Input: part model. Units: mm. Frame: model coordinates. A direction names the side the tool comes from. Give positions to 0.01 mm unless a question says otherwise; leave off trailing zeros. Order: outer loops, then holes, each group sorted by start corner. A loop starts at its lowest first (then second) coordinate and runs counter-clockwise, first axis right, second up. Notation, with made-up numbers: M 79,41 L 91,41 A16 ccw 91,66 Z; hole C 67,12.25 d6. An arc over 180 degrees is marked long. Use a Markdown table: item, result.
Autodesk Inventor part; units mm, degrees
ref_plane "YZ Plane" through (0, 0, 0) normal (1, 0, 0) x (0, 1, 0)
ref_plane "XZ Plane" through (0, 0, 0) normal (0, 1, 0) x (-1, 0, 0)
ref_plane "XY Plane" through (0, 0, 0) normal (0, 0, 1) x (1, 0, 0)
sketch "main" plane through (0, 0, 0) normal (0, 0, 1) x (1, 0, 0)
  circle A0 centre (13.5257, -15.1463) radius 2.1844
  circle A1 centre (-37.2743, -15.1463) radius 2.1844
  arc A2 (13.5257, -21.4963) -> (19.8757, -15.1463) centre (13.5257, -15.1463) ccw
  arc A3 (-37.2743, -8.7963) -> (-37.2743, -21.4963) centre (-37.2743, -15.1463) ccw
  line L0 (7.1757, 10.2537) -> (7.1757, 3.9037)
  line L1 (-5.5243, -8.7963) -> (-37.2743, -8.7963)
  arc A4 (-5.5243, -8.7963) -> (7.1757, 3.9037) centre (-5.5243, 3.9037) ccw
  line L2 (19.8757, 13.4287) -> (19.8757, -15.1463)
  line L3 (13.5257, -21.4963) -> (-37.2743, -21.4963)
  line L4 (10.3507, 13.4287) -> (19.8757, 13.4287)
  arc A5 (10.3507, 13.4287) -> (7.1757, 10.2537) centre (10.3507, 10.2537) ccw
  point P0 (6.3402, -4.1174)
  dimension "d0" = 12.7
  dimension "d1" = 12.7
  dimension "d2" = 12.7
  dimension "d5" = 50.8
  dimension "d7" = 34.925
  dimension "d8" = 3.175
sketch "Sketch1" plane through (0, 0, 0) normal (0, 1, 0) x (-1, 0, 0)
  circle A0 centre (0, 0) radius 2.1844
  circle A1 centre (-50.8, 0) radius 2.1844
  arc A2 (0, -6.35) -> (6.35, 0) centre (0, 0) ccw
  arc A3 (-50.8, 6.35) -> (-50.8, -6.35) centre (-50.8, 0) ccw
  line L0 (-6.35, 25.4) -> (-6.35, 19.05)
  line L1 (-19.05, 6.35) -> (-50.8, 6.35)
  arc A4 (-19.05, 6.35) -> (-6.35, 19.05) centre (-19.05, 19.05) ccw
  line L2 (6.35, 28.575) -> (6.35, 0)
  line L3 (0, -6.35) -> (-50.8, -6.35)
  line L4 (-3.175, 28.575) -> (6.35, 28.575)
  arc A5 (-3.175, 28.575) -> (-6.35, 25.4) centre (-3.175, 25.4) ccw
extrude "Extrusion1" add sketch "Sketch1" along normal blind 1.5875
properties part number "Magazine Gusset"
1) Mould query, pull axis Z, two halves, no side actions, for faces 3 (the face through (19, 1.588, 4)), 4 (the face through (-4.54, 0.78, -4.44)), 5 (the face through (48.716, 0.783, -0.656)), 6 (the face through (9.97, 0.78, 10.17)). Classes: released by +Z, released by -Z, zero draft, split by the parting line, or undercut.
Response values:
| item | result |
|---|---|
| face 3 | zero draft |
| face 4 | released by -Z |
| face 5 | undercut |
| face 6 | released by +Z |
2) Material intervals for line 1 (X direction, y = 0.7, z = -0.5); line 2 (Z direction, x = 50.8, y = 0.5); line 3 (Z direction, x = 32, y = 0.9), sorted ascending. Write a range as from..to.
Response values:
| item | result |
|---|---|
| line 1 | x = -6.33..-2.13, 2.13..48.67, 52.93..57.13 |
| line 2 | z = -6.35..-2.18, 2.18..6.35 |
| line 3 | z = -6.35..6.35 |
3) Cut plane A-A on y = 0.6. Return loops of the section in (x, z) (3 decimals).
Response values:
| item | result |
|---|---|
| outline | M -6.35,0 A6.35 ccw 0,-6.35 L 50.8,-6.35 A6.35 ccw 50.8,6.35 L 19.05,6.35 A12.7 cw 6.35,19.05 L 6.35,25.4 A3.175 ccw 3.175,28.575 L -6.35,28.575 Z; hole C 0,0 d4.369; hole C 50.8,0 d4.369 |
4) Cut plane C-C on z = 24. Return loops of the section in (x, y).
Response values:
| item | result |
|---|---|
| outline | M -6.35,0 L 6.35,0 L 6.35,1.59 L -6.35,1.59 Z |
5) Reachability of faces 1 (the face through (6.35, 1, 22)), 2 (the face through (-2.084, 0.783, -0.656)) from +Z, -Z, +X, -X, +Y, -Y: full face, straight path, thin tool, end or side. Return the list, or none.
Response values:
| item | result |
|---|---|
| face 1 | +Z, +X, +Y, -Y |
| face 2 | +Y, -Y |
6) Cut plane B-B on x = 33.5. Return loops of the section in (y, z), and give its area (3 significant figures).
Response values:
| item | result |
|---|---|
| outline | M 0,-6.35 L 1.59,-6.35 L 1.59,6.35 L 0,6.35 Z |
| area | 20.2 mm² |
7) First-contact query: pin 1 Ø0.8 at (y, z) = (1, 21.5) entering from +X; pin 2 Ø5 at (x, z) = (50.8, 0) entering from +Y; pin 3 Ø0.5 at (x, y) = (28.5, 1) entering from +Z; pin 4 Ø4 at (x, z) = (0, 0) entering from +Y. Flat tips, straight axial feed; report the tip coordinate or a pass-through.
Response values:
| item | result |
|---|---|
| pin 1 | stops at x = 6.35 |
| pin 2 | stops at y = 1.59 |
| pin 3 | stops at z = 6.35 |
| pin 4 | passes through |
